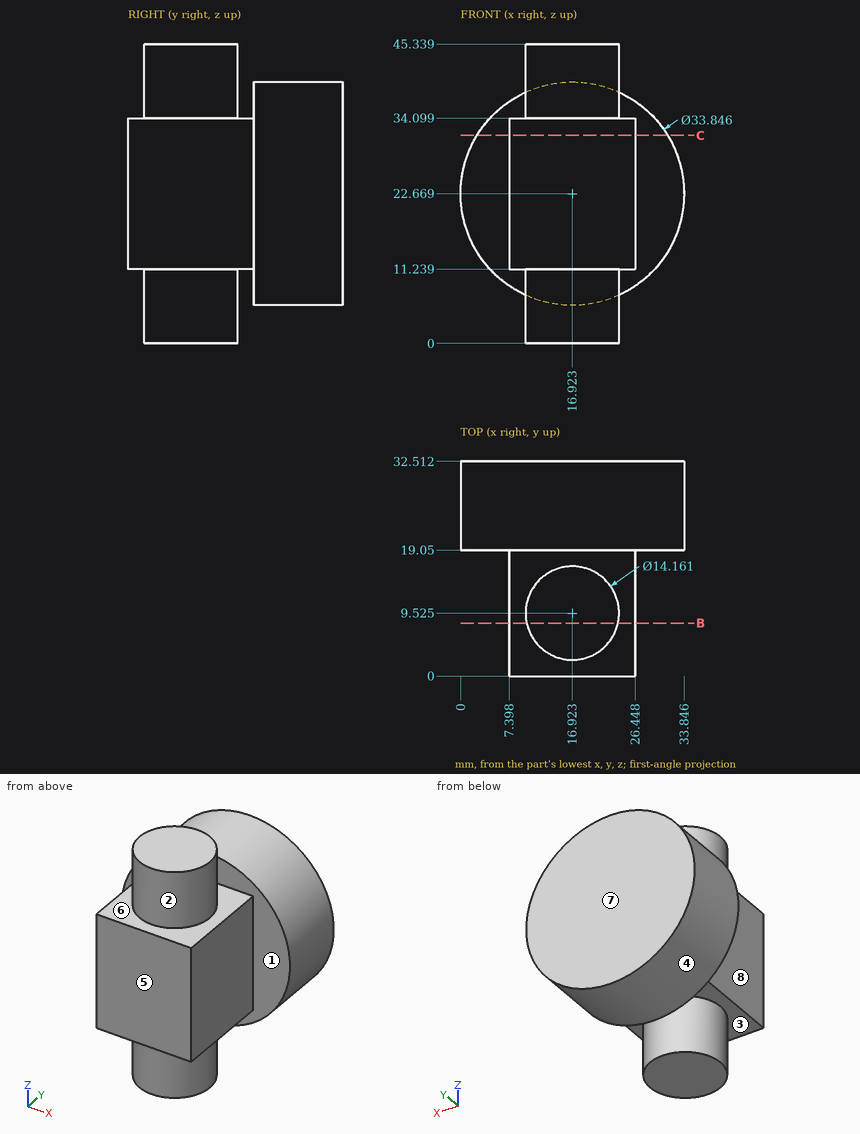
Job drawing, mm, ordinate dimensions from the low corner. One solid piece. A direction names the side the tool comes from. Coordinates: 2 decimals unless noted, no trailing zeros. Write each loop counter-clockwise with the first axis right and the second up, starting at its lowest first coordinate (ties: lowest second). Pieces come first, ordered by that corner, then holes. Notation, with made-up numbers: (73, 67.25) - (110, 67.25) arc R22 cw to (110, 106.25) - close; hole circle Ø7 at (31, 53.25). An arc over 180 degrees is marked (long way). Use a Markdown table: item, result. Add a question column.
Item 1: Mould opens along Y. For the marked faces 5, 6, 7 and 8 say: pulls with the +Y half, pulls with the -Y half, needs draft (parallel to the pull), parting line crosses it, or undercut.
Item 2: 3-axis set-ups, long thin cutter, end or side, ignore diameter. For the marked faces 1, 2, 3 and 4: which of +Z, -Z, +X, -X, +Y, -Y reach the whole face in a straight line?
Item 3: Drill centre lines: L1, parallel to Z at x = 17, y = 28; L2, parallel to X at y = 5.5, z = 12.5; L3, parallel to Y at x = 14.5, z = 38.5. Where is each one in solid material? Low to high. Write a range as from..to.
Item 4: Band-saw the part on C-C, the plane z = 31.5. Give the cut face in (x, y).
Item 5: Band-saw the part on B-B, the plane y = 8. Give the cut face in (x, z).
Item 6: Flat gauge pins, fed straight in: pin 1 (1.5 mm diameter, centred on x = 23.5, z = 10, fed in from -Y) (1 decimal); pin 2 (9.5 mm diameter, centred on x = 12, y = 11.5, fed in from -Z); pin 3 (8 mm diameter, centred on y = 20, z = 35, fed in from +X); pin 4 (9.5 mm diameter, centred on y = 11, z = 23, fed in from +X). Where does each tip first touch, or does it go through?
Numbers:
| question | item | result |
|---|---|---|
| 1 | face 5 | pulls with the -Y half |
| 1 | face 6 | undercut |
| 1 | face 7 | pulls with the +Y half |
| 1 | face 8 | needs draft |
| 2 | face 1 | none |
| 2 | face 2 | +Z |
| 2 | face 3 | -Z |
| 2 | face 4 | +Y |
| 3 | L1 | 5.75..39.59 |
| 3 | L2 | 7.4..26.45 |
| 3 | L3 | 2.87..16.18, 19.05..32.51 |
| 4 | outline | (2.49, 19.05) - (7.4, 19.05) - (7.4, 0) - (26.45, 0) - (26.45, 19.05) - (31.36, 19.05) - (31.36, 32.51) - (2.49, 32.51) - close |
| 5 | outline | (7.4, 11.24) - (10.01, 11.24) - (10.01, 0) - (23.84, 0) - (23.84, 11.24) - (26.45, 11.24) - (26.45, 34.1) - (23.84, 34.1) - (23.84, 45.34) - (10.01, 45.34) - (10.01, 34.1) - (7.4, 34.1) - close |
| 6 | pin 1 | y = 5.5 |
| 6 | pin 2 | z = 0 |
| 6 | pin 3 | x = 31.65 |
| 6 | pin 4 | x = 26.45 |
